Autodesk Inventor part; units mm, degrees
ref_plane "YZ Plane" through (0, 0, 0) normal (1, 0, 0) x (0, 1, 0)
ref_plane "XZ Plane" through (0, 0, 0) normal (0, 1, 0) x (-1, 0, 0)
ref_plane "XY Plane" through (0, 0, 0) normal (0, 0, 1) x (1, 0, 0)
sketch "Sketch1" plane through (0, 0, 0) normal (0, 1, 0) x (-1, 0, 0)
  line L0 (-54.9089, 0) -> (-54.9089, -19.92)
  line L1 (-0.4496, -19.92) -> (-0.4496, 0)
  circle A0 centre (-74.4786, -9.96) radius 3.6
  circle A1 centre (-81.4786, -9.96) radius 1.05
  circle A2 centre (-74.4786, -16.96) radius 1.05
  circle A3 centre (-67.4786, -9.96) radius 1.05
  circle A4 centre (-74.4786, -2.96) radius 1.05
  circle A5 centre (19.12, -9.96) radius 2.6
  circle A6 centre (26.12, -9.96) radius 1.05
  circle A7 centre (19.12, -16.96) radius 1.05
  circle A8 centre (12.12, -9.96) radius 1.05
  circle A9 centre (19.12, -2.96) radius 1.05
  circle A10 centre (-42.6793, -39.96) radius 1.55
  circle A11 centre (-27.6793, -39.96) radius 1.55
  circle A12 centre (-12.6793, -39.96) radius 1.55
  arc A13 (19.19, -19.92) -> (19.19, 0) centre (19.19, -9.96) ccw
  line L2 (19.19, -19.92) -> (-0.8993, -19.92)
  arc A14 (-74.5486, 0) -> (-74.5486, -19.92) centre (-74.5486, -9.96) ccw
  line L3 (-54.4593, -19.92) -> (-74.5486, -19.92)
  line L4 (-54.4593, -50) -> (-54.4593, -19.92)
  line L5 (-0.8993, -19.92) -> (-0.8993, -50)
  line L6 (-0.8993, -50) -> (-54.4593, -50)
  line L7 (-74.5486, 0) -> (19.19, 0)
  line L8 (-55.3586, -19.92) -> (-55.3586, 0)
  line L9 (-54.4593, 0) -> (-54.4593, -19.92)
  line L10 (-0.8993, -19.92) -> (-0.8993, 0)
  line L11 (0, 0) -> (0, -19.92)
extrude "Extrusion1" add sketch "Sketch1" against normal blind 1.5
properties part number "axis_23_bottom_frame"
The model under review builds one solid part; all positions refer to its coordinate system, in mm. Round coordinates to 2 decimals unless told otherwise and drop trailing zeros. Loops run counter-clockwise (first coordinate to the right, second up) from the corner with the lowest first, then second, coordinate; pieces in that order, holes last. Notation, with made-up numbers: (-0.5, -31.5) -> (10.5, -31.5) arc R15 cw to (10.5, -19.5) -> close; hole circle Ø5 at (50, 80). An arc over 180 degrees is marked (long way). Answer as a JSON object with one key per item and string values. Group by question number.
1) We need section C-C on z = -16.96. Write out the cut boundary in (x, y).
2) For pin 1 Ø1.9 at (x, z) = (-12.12, -9.96) entering from -Y; pin 2 Ø0.8 at (y, z) = (-0.5, -36.5) entering from +X; pin 3 Ø0.8 at (y, z) = (-0.5, -34.5) entering from -X; pin 4 Ø0.8 at (x, y) = (66.5, -1) entering from -Z, all flat-tipped, find the tip position at first contact; note any pin that passes through.
3) We need section A-A on x = -12.12. Write out the cut boundary in (y, z), then the cut area to 3 significant figures.
4) We need section B-B on y = -0.25. Give the number of separate pieces and of enclosed holes in the cut face, then the cut area to 3 significant figures.
5) For line 1 (Z direction, x = -19.12, y = -0.8); line 2 (X direction, y = -0.05, z = -17.5); line 3 (Z direction, x = 64.5, y = -0.05), list the stretches that pass through material, from the lowest coordinate up. Write a range as [from, to].
6) Mouldability with a two-part tool opening along Z and no side actions: class faces 1 (the face through (28.015, -0.74, -41.473)), 2 (the face through (28, 0, -19)), 3 (the face through (84.506, -0.74, -9.741)) as released by +Z, released by -Z, zero draft, split by the parting line, or undercut.
7) We need section D-D on x = -26.12. Write out the cut boundary in (y, z).
Result set:
{
 "1": {"outline": "(-26.28, -1.5) -> (-20.17, -1.5) -> (-20.17, 0) -> (-26.28, 0) -> close; (-18.07, -1.5) -> (73.43, -1.5) -> (73.43, 0) -> (-18.07, 0) -> close; (75.53, -1.5) -> (81.63, -1.5) -> (81.63, 0) -> (75.53, 0) -> close"},
 "2": {"pin 1": "through", "pin 2": "x = 54.46", "pin 3": "x = 0.9", "pin 4": "z = -19.92"},
 "3": {"outline": "(-1.5, -19.92) -> (0, -19.92) -> (0, -11.01) -> (-1.5, -11.01) -> close; (-1.5, -8.91) -> (0, -8.91) -> (0, 0) -> (-1.5, 0) -> close", "area": "26.7 mm²"},
 "4": {"separate pieces": "1", "enclosed holes": "13", "area": "3,680 mm²"},
 "5": {"line 1": "[-19.92, -18.01], [-15.91, -12.56], [-7.36, -4.01], [-1.91, 0]", "line 2": "[-25.7, -20.02], [-18.22, 73.58], [75.38, 81.06]", "line 3": "[-19.92, 0]"},
 "6": {"face 1": "undercut", "face 2": "zero draft", "face 3": "split by the parting line"},
 "7": {"outline": "(-1.5, -17.11) -> (0, -17.11) -> (0, -11.01) -> (-1.5, -11.01) -> close; (-1.5, -8.91) -> (0, -8.91) -> (0, -2.81) -> (-1.5, -2.81) -> close"}
}
